Could you check a few things on this model? Use its own coordinates, in mm. Coordinates: 2 decimals unless noted, no trailing zeros. Write each loop counter-clockwise with the first axis right and the second up, starting at its lowest first coordinate (ties: lowest second). Pieces come first, ordered by that corner, then holes. Notation, with made-up numbers: (-36, 68) - (-11, 68) arc R21 ccw to (-11, 72) - close; hole circle Ø8 at (-21.75, 79.25). An arc over 180 degrees is marked (long way). Write item = value, one per line. Start each with the question number.
```python
from build123d import *

# Parameters (mm, degrees)
F0_W          = 1300
F0_H          = 340
F1_DEPTH      = 13
F2_T          = -0.9
F3_W          = 724
F3_H          = 273
F4_DEPTH      = 0.901
F4_DEPTH_BACK = 12.101
F5_R          = 75
F6_DEPTH      = 12.101
F6_DEPTH_BACK = 0.901


with BuildPart() as f1:
    # F0 (on Top) → F1 (new body)
    with BuildSketch(Plane.XY):
        Rectangle(F0_W, F0_H)
    extrude(amount=F1_DEPTH)

    # F2
    f2_openings = [f1.faces().sort_by_distance(p)[0] for p in [
        (0, 0, 13),
    ]]
    offset(amount=F2_T, openings=f2_openings)

    # F3 (on face) → F4 (cut, two sides)
    with BuildSketch(Plane.XY.offset(0.9)) as f4_sk:
        with Locations((0, 6.5)):
            Rectangle(F3_W, F3_H)
    extrude(amount=-F4_DEPTH, mode=Mode.SUBTRACT)
    extrude(f4_sk.sketch, amount=-F4_DEPTH_BACK, mode=Mode.SUBTRACT)

    # F5 (on face) → F6 (cut, two sides)
    with BuildSketch(Plane.XY.offset(0.9)) as f6_sk:
        with Locations((-518, 6.5)):
            Circle(F5_R)
        with Locations((518, 6.5)):
            Circle(F5_R)
    extrude(amount=F6_DEPTH, mode=Mode.SUBTRACT)
    extrude(f6_sk.sketch, amount=-F6_DEPTH_BACK, mode=Mode.SUBTRACT)


solid = f1.part
```
1) Suppose I cut it at C-C on y = 119.5. Please give me the cut outline in (x, z), plus the area to 3 significant figures.
2) Suppose I cut it at A-A on x = 245. Please give me the cut outline in (y, z), plus the area to 3 significant figures.
3) Suppose I cut it at D-D on y = 6.5. Please give me the cut outline in (x, z).
4) Suppose I cut it at B-B on z = 4.25. Please give me the cut outline in (x, y), plus the area to 3 significant figures.
5) If I drill on probe 1 along Y at (x, z) = (-577.5, 3); probe 2 along X at (y, z) = (-76, 3); probe 3 along Y at (x, z) = (518, 0.75), over which ranges is the centre line in solid material (lowest first)? Write a range as [from, to].
6) For P1, Ø2, axis at x = 445.5, y = 68.5, coming from the +Z side, with a flat end and sliding along its axis, tell me the tip position at first contact or that it passes through.
7) Thinking about a two-plate mould opening in X: for faces 1 (the flat face through (-9, -148, 0.9)), 2 (the flat face through (-9, -149, 0)), 3 (the cylindrical face through (-448.72, -22.23, 0.46)), which applies, +X half, -X half, draft (parallel to the pull), parting line (faces both ways), or undercut?
Reply:
q1.outline = (-650, 0) - (-362, 0) - (-362, 0.9) - (-649.1, 0.9) - (-649.1, 13) - (-650, 13) - close; (362, 0) - (650, 0) - (650, 13) - (649.1, 13) - (649.1, 0.9) - (362, 0.9) - close
q1.area = 540 mm^2
q2.outline = (-170, 0) - (-130, 0) - (-130, 0.9) - (-169.1, 0.9) - (-169.1, 13) - (-170, 13) - close; (143, 0) - (170, 0) - (170, 13) - (169.1, 13) - (169.1, 0.9) - (143, 0.9) - close
q2.area = 82.1 mm^2
q3.outline = (-650, 0) - (-593, 0) - (-593, 0.9) - (-649.1, 0.9) - (-649.1, 13) - (-650, 13) - close; (-443, 0) - (-362, 0) - (-362, 0.9) - (-443, 0.9) - close; (362, 0) - (443, 0) - (443, 0.9) - (362, 0.9) - close; (593, 0) - (650, 0) - (650, 13) - (649.1, 13) - (649.1, 0.9) - (593, 0.9) - close
q4.outline = (-650, -170) - (650, -170) - (650, 170) - (-650, 170) - close; hole (-649.1, -169.1) - (649.1, -169.1) - (649.1, 169.1) - (-649.1, 169.1) - close
q4.area = 2,950 mm^2
q5.probe_1 = [-170, -169.1], [169.1, 170]
q5.probe_2 = [-650, -649.1], [649.1, 650]
q5.probe_3 = [-170, -68.5], [81.5, 170]
q6.P1 = 0.9
q7.face_1 = undercut
q7.face_2 = draft
q7.face_3 = undercut
